For this review, take the finished solid that the model builds, in its own axes (mm). A direction names the side the tool comes from. Round coordinates to 2 decimals unless told otherwise and drop trailing zeros. Loops run counter-clockwise (first coordinate to the right, second up) from the corner with the lowest first, then second, coordinate; pieces in that order, holes last. Notation, with made-up numbers: (32.25, -20.75) -> (50.25, -20.75) arc R26 ccw to (50.25, 14.25) -> close; hole circle Ø8 at (76, 63). An arc over 180 degrees is marked (long way). One line per question, with ' | ' between items. Start each with the question number.
1. Consider section D-D (z = 36.5). Write out the cut boundary in (x, y).
2. For pin 1 Ø1.2 at (x, z) = (15, 106.5) entering from -Y; pin 2 Ø1.5 at (x, y) = (9, 19.5) entering from +Z; pin 3 Ø6 at (y, z) = (2, 56) entering from -X; pin 4 Ø2 at (x, z) = (14, 65) entering from -Y, all flat-tipped, find the tip position at first contact; note any pin that passes through.
3. Consider section C-C (y = 8). Write out the cut boundary in (x, z).
4. Consider section A-A (z = 106.2). Write out the cut boundary in (x, y), and give its area (3 significant figures).
5. For faces 1 (the face through (-15.15, -12.51, 69.54)), 2 (the face through (-2.018, 15.368, 28.2)), 3 (the face through (0, -13, 57.2)), 4 (the face through (16, -13.5, 108)), 5 (the face through (-3.4, 17.8, 94.4)), list the 3-axis set-ups (+Z, -Z, +X, -X, +Y, -Y) from which the entire face can be reached by the end or side of a thin tool; tool diameter is ignored.
6. Consider section B-B (y = 0). Write out the cut boundary in (x, z), and give its area (3 significant figures).
7. Wall thickness on line 1 along X through (y, z) = (-9, 106); line 2 along Z through (x, y) = (14, -11); line 3 along Z through (x, y) = (-14, -6): over which ranges is each line inside the solid? List them lowest first.
8. Draft analysis for pull direction X (two halves, no side actions). For faces 6 (the face through (14, -4.5, 66)), 7 (the face through (0.35, 16.63, 86.55)), 8 (the face through (0, 2, 115.2)), 9 (the face through (14.188, -9.063, 108.198)), state which applies: pulls with the +X half, pulls with the -X half, needs draft (parallel to the pull), parting line crosses it, or undercut.
```python
from build123d import *

# Parameters (mm, degrees)
SZKIC1_R                    = 15.5
DODANIE_WYCI_GNI_CIE1_DEPTH = 57.2
SZKIC2_W                    = 40.2
SZKIC2_H                    = 27
DODANIE_WYCI_GNI_CIE2_DEPTH = 58
SZKIC3_R                    = 8
DODANIE_WYCI_GNI_CIE3_DEPTH = 2.3
SZKIC4_R                    = 3
DODANIE_WYCI_GNI_CIE4_DEPTH = 14.7
SZKIC5_W                    = 6.794003974
SZKIC5_H                    = 1.284090098
WYTNIJ_WYCI_GNI_CIE1_DEPTH  = 13
SZKIC6_R                    = 2
WYTNIJ_WYCI_GNI_CIE2_DEPTH  = 7
SZKIC7_R                    = 9.25
DODANIE_WYCI_GNI_CIE5_DEPTH = 4.5
DODANIE_WYCI_GNI_CIE6_START = 2
SZKIC8_R                    = 3.5
SZKIC8_R_2                  = 2
DODANIE_WYCI_GNI_CIE6_DEPTH = 2


with BuildPart() as part:
    # Szkic1 → Dodanie-wyciągnięcie1 (new body)
    with BuildSketch(Plane.XY):
        Circle(SZKIC1_R)
    extrude(amount=DODANIE_WYCI_GNI_CIE1_DEPTH)

    # Szkic2 → Dodanie-wyciągnięcie2 (add)
    with BuildSketch(Plane.XY.offset(57.2)):
        with Locations((0, 2)):
            Rectangle(SZKIC2_W, SZKIC2_H)
    extrude(amount=DODANIE_WYCI_GNI_CIE2_DEPTH)

    # Szkic3 → Dodanie-wyciągnięcie3 (add)
    with BuildSketch(Plane(origin=(0, 15.5, 0), x_dir=(1, 0, 0), z_dir=(0, 1, 0))):
        with Locations(Location((0, -94.540551958, 0), (0, 0, 270))):
            Circle(SZKIC3_R)
    extrude(amount=DODANIE_WYCI_GNI_CIE3_DEPTH)

    # Szkic4 → Dodanie-wyciągnięcie4 (add)
    with BuildSketch(Plane(origin=(0, 17.8, 0), x_dir=(1, 0, 0), z_dir=(0, 1, 0))):
        with Locations(Location((0, -94.540551958, 0), (0, 0, 270))):
            Circle(SZKIC4_R)
    extrude(amount=DODANIE_WYCI_GNI_CIE4_DEPTH)

    # Szkic5 → Wytnij-wyciągnięcie1 (cut)
    with BuildSketch(Plane(origin=(0, 32.5, 0), x_dir=(1, 0, 0), z_dir=(0, 1, 0))):
        with Locations((0.179126758, -96.898506909)):
            Rectangle(SZKIC5_W, SZKIC5_H)
    extrude(amount=-WYTNIJ_WYCI_GNI_CIE1_DEPTH, mode=Mode.SUBTRACT)

    # Szkic6 → Wytnij-wyciągnięcie2 (cut)
    with BuildSketch(Plane.XZ.offset(11.5)):
        with Locations(Location((14.1, 106.2, 0), (0, 0, 270))):
            Circle(SZKIC6_R)
        with Locations(Location((14.1, 66.2, 0), (0, 0, 90))):
            Circle(SZKIC6_R)
        with Locations(Location((-14.1, 66.2, 0), (0, 0, 270))):
            Circle(SZKIC6_R)
        with Locations(Location((-14.1, 106.2, 0), (0, 0, 90))):
            Circle(SZKIC6_R)
    extrude(amount=-WYTNIJ_WYCI_GNI_CIE2_DEPTH, mode=Mode.SUBTRACT)

    # Szkic7 → Dodanie-wyciągnięcie5 (add)
    with BuildSketch(Plane.XZ.offset(11.5)):
        with Locations(Location((0, 95.2, 0), (0, 0, 90))):
            Circle(SZKIC7_R)
    extrude(amount=DODANIE_WYCI_GNI_CIE5_DEPTH)

    # Szkic8 → Dodanie-wyciągnięcie6 (add)
    # profile 1 of 4: a face of its own
    with BuildSketch(Plane.XZ.offset(11.5).offset(DODANIE_WYCI_GNI_CIE6_START)):
        with Locations(Location((14.1, 106.2, 0), (0, 0, 90))):
            Circle(SZKIC8_R)
        with Locations(Location((14.1, 106.2, 0), (0, 0, 270))):
            Circle(SZKIC8_R_2, mode=Mode.SUBTRACT)
    # profile 2 of 4: a face of its own
    with BuildSketch(Plane.XZ.offset(11.5).offset(DODANIE_WYCI_GNI_CIE6_START)):
        with Locations(Location((14.1, 66.2, 0), (0, 0, 90))):
            Circle(SZKIC8_R)
        with Locations(Location((14.1, 66.2, 0), (0, 0, 270))):
            Circle(SZKIC8_R_2, mode=Mode.SUBTRACT)
    # profile 3 of 4: a face of its own
    with BuildSketch(Plane.XZ.offset(11.5).offset(DODANIE_WYCI_GNI_CIE6_START)):
        with Locations(Location((-14.1, 66.2, 0), (0, 0, 90))):
            Circle(SZKIC8_R)
        with Locations(Location((-14.1, 66.2, 0), (0, 0, 270))):
            Circle(SZKIC8_R_2, mode=Mode.SUBTRACT)
    # profile 4 of 4: a face of its own
    with BuildSketch(Plane.XZ.offset(11.5).offset(DODANIE_WYCI_GNI_CIE6_START)):
        with Locations(Location((-14.1, 106.2, 0), (0, 0, 90))):
            Circle(SZKIC8_R)
        with Locations(Location((-14.1, 106.2, 0), (0, 0, 270))):
            Circle(SZKIC8_R_2, mode=Mode.SUBTRACT)
    extrude(amount=-DODANIE_WYCI_GNI_CIE6_DEPTH)


solid = part.part
```
Answer block:
1) outline: circle Ø31 at (0, 0)
2) pin 1: stops at y = -4.5 | pin 2: passes through | pin 3: stops at x = -20.1 | pin 4: stops at y = -13.5
3) outline: (-20.1, 57.2) -> (-13.28, 57.2) -> (-13.28, 0) -> (13.28, 0) -> (13.28, 57.2) -> (20.1, 57.2) -> (20.1, 115.2) -> (-20.1, 115.2) -> close
4) outline: (-20.1, -11.5) -> (-17.6, -11.5) -> (-17.6, -13.5) -> (-16.1, -13.5) -> (-16.1, -4.5) -> (-12.1, -4.5) -> (-12.1, -13.5) -> (-10.6, -13.5) -> (-10.6, -11.5) -> (10.6, -11.5) -> (10.6, -13.5) -> (12.1, -13.5) -> (12.1, -4.5) -> (16.1, -4.5) -> (16.1, -13.5) -> (17.6, -13.5) -> (17.6, -11.5) -> (20.1, -11.5) -> (20.1, 15.5) -> (-20.1, 15.5) -> close | area: 1,040 mm2
5) face 1: -Y | face 2: -Z | face 3: +X, -X, -Y | face 4: +Z, -Z, +X, -Y | face 5: +Y
6) outline: (-20.1, 57.2) -> (-15.5, 57.2) -> (-15.5, 0) -> (15.5, 0) -> (15.5, 57.2) -> (20.1, 57.2) -> (20.1, 115.2) -> (-20.1, 115.2) -> close | area: 4,100 mm2
7) line 1: x = -20.1 to -16.09, -12.11 to 12.11, 16.09 to 20.1 | line 2: z = 57.2 to 64.2, 68.2 to 104.2, 108.2 to 115.2 | line 3: z = 0 to 64.2, 68.2 to 104.2, 108.2 to 115.2
8) face 6: undercut | face 7: parting line crosses it | face 8: needs draft | face 9: undercut
